Here's how the part is built. I have some questions about the finished solid (model axes, mm). A direction names the side the tool comes from. Coordinates: 2 decimals unless noted, no trailing zeros. Order: outer loops, then holes, each group sorted by start corner. A loop starts at its lowest first (then second) coordinate and runs counter-clockwise, first axis right, second up. Notation, with made-up numbers: (16, 55) - (38, 55) arc R10 cw to (38, 74) - close; hole circle Ø8 at (2, -35). An arc over 180 degrees is marked (long way). Answer in a Markdown table with one row per item. Add a question column.
Item 1: On a 3-axis mill with a long thin cutter (end or side, diameter ignored), from which of +Z, -Z, +X, -X, +Y, -Y can I reach the whole of each face in a straight line? I mean faces 1 (the flat face through (25, 20, 0)), 2 (the cylindrical face through (-12.2, 4.25, -34.92)), 3 (the flat face through (38.75, 8.8, 10.8)), 4 (the flat face through (32.75, 15, 5)). Say none if no direction works.
Item 2: I want a section at B-B (y = 11.5). Please give me the cut outline in (x, z), plus the area to 3 significant figures.
Item 3: If I drill on line 1 along X through (y, z) = (20, 6.5); line 2 along X through (y, z) = (27.5, -5); line 3 along Z through (x, y) = (40, 10), over which ranges is the centre line in solid material (lowest first)? Write a range as from..to.
Item 4: I want a section at A-A (z = -35). Please give me the cut outline in (x, y), plus the area to 3 significant figures.
Item 5: Thinking about a two-plate mould opening in Z: for faces 5 (the flat face through (37.25, 16, 5)), 6 (the flat face through (15, 5, 15)), 7 (the flat face through (-5, 16, -37.25)), 8 (the cylindrical face through (-5.07, 25.25, -34.95)), which applies, +Z half, -Z half, draft (parallel to the pull), parting line (faces both ways), or undercut?
Item 6: I want a section at C-C (x = -4). Please give me the cut outline in (y, z).
Item 7: I want a section at D-D (z = 3.5). Please give me the cut outline in (x, y), plus the area to 3 significant figures.
Item 8: Will these pins go through, and if not, where does the flat tip stop? pin 1 Ø8 at (x, y) = (-4.5, 17) entering from +Z; pin 2 Ø10.5 at (y, z) = (15, -9.5) entering from -X; pin 3 Ø12 at (y, z) = (35, -20.5) entering from +X.
```python
from build123d import *

# Parameters (mm, degrees)
BOSS_EXTRUDE1_DEPTH = 40
BOSS_EXTRUDE2_DEPTH = 15
DRAFT1_START        = -20
DRAFT1_DEPTH        = 70
DRAFT1_START_2      = -50
DRAFT1_2_DEPTH      = 71
CUT_EXTRUDE1_DEPTH  = 88.749643874
CUT_EXTRUDE3_DEPTH  = 88.749643874


with BuildPart() as part:
    # Sketch1 → Boss-Extrude1 (new body)
    with BuildSketch(Plane(origin=(0, 0, 0), x_dir=(1, 0, 0), z_dir=(0, 1, 0))):
        Polygon((0, 0), (0, 50), (-10, 50), (-10, -10), (50, -10), (50, 0), align=None)
    extrude(amount=BOSS_EXTRUDE1_DEPTH)

    # Sketch2 → Boss-Extrude2 (add)
    with BuildSketch(Plane.XZ):
        Polygon((50, 20), (50, 10), (-10, 10), (-10, -50), (-20, -50), (-20, 20), align=None)
    extrude(amount=-BOSS_EXTRUDE2_DEPTH)

    # Draft1: read off the stored shape, not the designer's step
    # Draft1 outline → Draft1 (cut)
    with BuildSketch(Plane.YZ.offset(DRAFT1_START)):
        Polygon((0, 20), (10, 10), (15, 10), (15, 20), align=None)
    extrude(amount=DRAFT1_DEPTH, mode=Mode.SUBTRACT)

    # Draft1 2 outline → Draft1 2 (cut)
    with BuildSketch(Plane.XY.offset(DRAFT1_START_2)):
        Polygon((-20, 0), (-10, 10), (-10, 15), (-20, 15), align=None)
    extrude(amount=DRAFT1_2_DEPTH, mode=Mode.SUBTRACT)

    # Sketch3 → Cut-Extrude1 (cut, through all)
    with BuildSketch(Plane.XY.offset(10)):
        with BuildLine():
            Line((37.25, 23), (37.25, 8))
            ThreePointArc((37.25, 8), (35, 5.75), (32.75, 8))
            Line((32.75, 8), (32.75, 23))
            ThreePointArc((32.75, 23), (35, 25.25), (37.25, 23))
        make_face()
    cut_extrude1 = extrude(amount=-CUT_EXTRUDE1_DEPTH, mode=Mode.SUBTRACT)

    # Sketch4 → Cut-Extrude3 (cut, through all)
    with BuildSketch(Plane.XY.offset(10)):
        with BuildLine():
            Line((38.75, 8), (38.75, 23))
            ThreePointArc((38.75, 23), (35, 26.75), (31.25, 23))
            Line((31.25, 23), (31.25, 8))
            ThreePointArc((31.25, 8), (35, 4.25), (38.75, 8))
        make_face()
    cut_extrude3 = extrude(amount=CUT_EXTRUDE3_DEPTH, mode=Mode.SUBTRACT)

    # Mirror1: Cut-Extrude1, Cut-Extrude3 across plane
    add(cut_extrude1.mirror(Plane(origin=(0, 0, 0), x_dir=(-0.7071067811865476, 0, 0.7071067811865476), z_dir=(-0.7071067811865477, 0, -0.7071067811865475))), mode=Mode.SUBTRACT)
    add(cut_extrude3.mirror(Plane(origin=(0, 0, 0), x_dir=(-0.7071067811865476, 0, 0.7071067811865476), z_dir=(-0.7071067811865477, 0, -0.7071067811865475))), mode=Mode.SUBTRACT)


solid = part.part
```
Values follow:
| question | item | result |
|---|---|---|
| 1 | face 1 | -Z, +X, +Y, -Y |
| 1 | face 2 | -X, +Y |
| 1 | face 3 | +Z, +Y |
| 1 | face 4 | +Z, -Z |
| 2 | outline | (-10, -50) - (0, -50) - (0, -37.25) - (-10, -37.25) - close; (-10, -32.75) - (0, -32.75) - (0, 0) - (32.75, 0) - (32.75, 10) - (-10, 10) - close; (37.25, 0) - (50, 0) - (50, 10) - (37.25, 10) - close |
| 2 | area | 1,010 mm^2 |
| 3 | line 1 | x = -10..32.75, 37.25..50 |
| 3 | line 2 | x = -10..0 |
| 3 | line 3 | z = 0..10 |
| 4 | outline | (-20, 0) - (0, 0) - (0, 5.75) - (-10, 5.75) - (-10, 4.25) - (-15.75, 4.25) - close; (-10, 25.25) - (0, 25.25) - (0, 40) - (-10, 40) - close |
| 4 | area | 238 mm^2 |
| 5 | face 5 | draft |
| 5 | face 6 | +Z half |
| 5 | face 7 | undercut |
| 5 | face 8 | undercut |
| 6 | outline | (0, -50) - (40, -50) - (40, 10) - (10, 10) - (0, 20) - close; hole (8, -37.25) - (23, -37.25) arc R2.25 ccw to (23, -32.75) - (8, -32.75) arc R2.25 ccw to start |
| 7 | outline | (-20, 0) - (50, 0) - (50, 40) - (-10, 40) - (-10, 10) - close; hole (32.75, 8) arc R2.25 ccw to (37.25, 8) - (37.25, 23) arc R2.25 ccw to (32.75, 23) - close |
| 7 | area | 2,370 mm^2 |
| 8 | pin 1 | stops at z = 10 |
| 8 | pin 2 | stops at x = -10.25 |
| 8 | pin 3 | stops at x = 0 |
